Input: dimensioned drawing with shaded views. Units: mm. Origin: part minimum x, y, z. A direction names the side the tool comes from. Give positions to 0.01 mm unless a question says otherwise; leave off trailing zeros. Write each loop counter-clockwise with the first axis right and the second up, starting at its lowest first coordinate (ties: lowest second). Pieces come first, ordered by that corner, then holes. Notation, with made-up numbers: (88.5, 39) - (117.5, 39) arc R30 cw to (117.5, 66) - close; hole circle Ø3 at (-9, -1.5). An arc over 180 degrees is marked (long way). Answer as CSV lines item,"result".
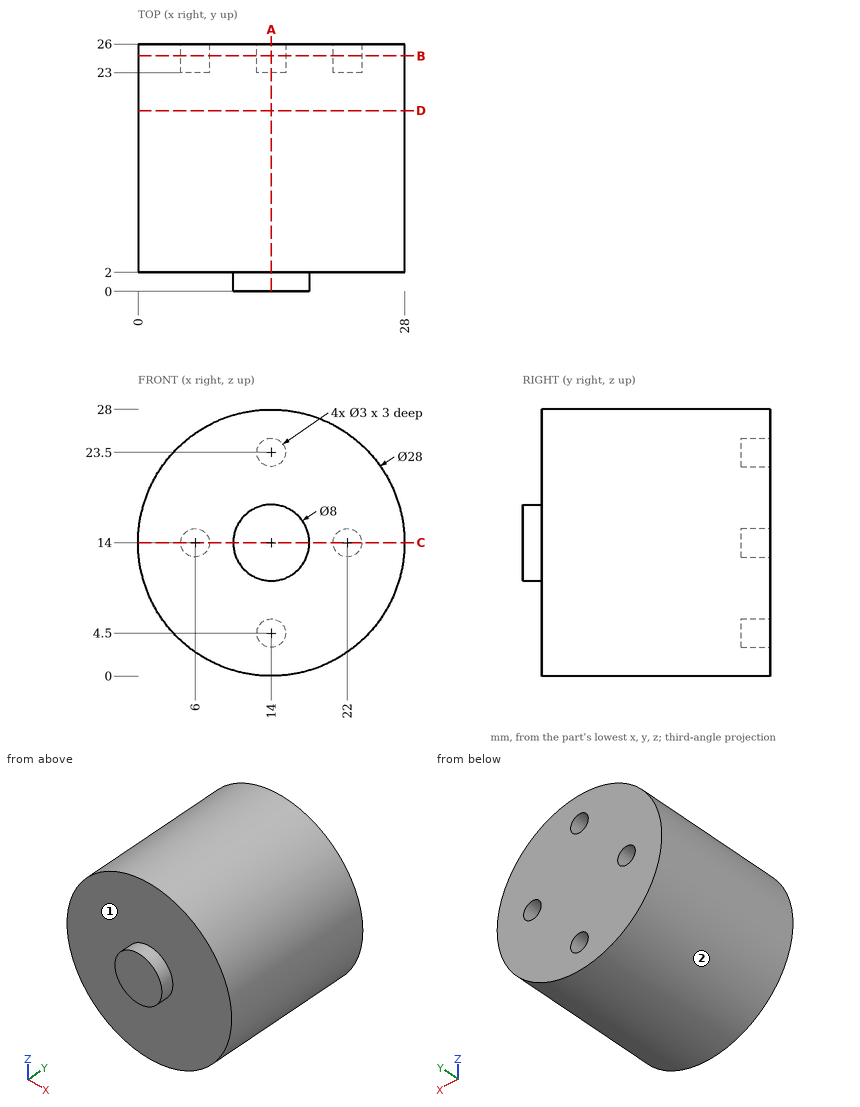
Item 1: Reachability of the marked faces 1 and 2 from +Z, -Z, +X, -X, +Y, -Y: full face, straight path, thin tool, end or side. Return the list, or none.
The answers:
face 1,"-Y"
face 2,"+Y, -Y"
Item 2: Cut plane A-A on x = 14. Return the cut outline in (y, z), plus the area to 3 significant figures.
The answers:
outline,"(0, 10) - (2, 10) - (2, 0) - (26, 0) - (26, 3) - (23, 3) - (23, 6) - (26, 6) - (26, 22) - (23, 22) - (23, 25) - (26, 25) - (26, 28) - (2, 28) - (2, 18) - (0, 18) - close"
area,"670 mm²"
Item 3: Cut plane B-B on y = 24.75. Return the cut outline in (x, z), plus the area to 3 significant figures.
The answers:
outline,"circle Ø28 at (14, 14); hole circle Ø3 at (6, 14); hole circle Ø3 at (14, 4.5); hole circle Ø3 at (14, 23.5); hole circle Ø3 at (22, 14)"
area,"587 mm²"
Item 4: Ray query, line 1 (Z direction, x = 14, y = 24.35); line 2 (X direction, y = 25.1, z = 14); line 3 (Y direction, x = 10, z = 10.5). Return the intervals inside material, ascending. Write a range as from..to.
The answers:
line 1,"0..3, 6..22, 25..28"
line 2,"0..4.5, 7.5..20.5, 23.5..28"
line 3,"2..26"
Item 5: Cut plane C-C on z = 14. Return the cut outline in (x, y), plus the area to 3 significant figures.
The answers:
outline,"(0, 2) - (10, 2) - (10, 0) - (18, 0) - (18, 2) - (28, 2) - (28, 26) - (23.5, 26) - (23.5, 23) - (20.5, 23) - (20.5, 26) - (7.5, 26) - (7.5, 23) - (4.5, 23) - (4.5, 26) - (0, 26) - close"
area,"670 mm²"
Item 6: Cut plane D-D on y = 19. Return the cut outline in (x, z).
The answers:
outline,"circle Ø28 at (14, 14)"
Item 7: Contact query for flat-ended pins moving along their axis: pin 1 (1 mm diameter, centred on y = 11, z = 16.5, fed in from +X); pin 2 (1.8 mm diameter, centred on x = 6, z = 14, fed in from +Y); pin 3 (12 mm diameter, centred on x = 22, z = 5.5, fed in from -Y). Output: stop coordinate, or through.
The answers:
pin 1,"x = 27.86"
pin 2,"y = 23"
pin 3,"y = 2"
